```python
from build123d import *

# Parameters (mm, degrees)
CUT_EXTRUDE_1_DEPTH = 2


with BuildPart() as part:
    # 草图1 → 旋转1 (revolve)
    with BuildSketch(Plane.XY, mode=Mode.PRIVATE) as revolve_1_sk:
        Polygon((0, 14), (-3, 14), (-1.25, 12.25), (-1.25, 11.25), (-1.5, 11.25), (-1.5, 0), (0, 0), align=None)
    revolve(revolve_1_sk.sketch.rotate(Axis((0, 0, 0), (0, 1, 0)), 270), axis=Axis((0, 0, 0), (0, 1, 0)))

    # 草图2 → 切除-拉伸1 (cut)
    with BuildSketch(Plane(origin=(0, 14, 0), x_dir=(1, 0, 0), z_dir=(0, 1, 0))):
        Polygon((0.577350269, 1), (-0.577350269, 1), (-1.154700538, 0), (-0.577350269, -1), (0.577350269, -1), (1.154700538, 0), align=None)
    extrude(amount=-CUT_EXTRUDE_1_DEPTH, mode=Mode.SUBTRACT)


solid = part.part
```
Work out the finished part from the listing and answer in its coordinate system (mm). A direction names the side the tool comes from. Round coordinates to 2 decimals unless told otherwise and drop trailing zeros. Loops run counter-clockwise (first coordinate to the right, second up) from the corner with the lowest first, then second, coordinate; pieces in that order, holes last. Notation, with made-up numbers: (47.25, -13) -> (55.25, -13) arc R30 cw to (55.25, 19) -> close; hole circle Ø10 at (-33.5, 1.25). An arc over 180 degrees is marked (long way). Write each question's results on one line, items separated by ' | '. Start each with the question number.
1. For a pull along Z with two mould halves and no side action, classify faces 1 (the face through (-0.86, 13.01, -0.51)), 2 (the face through (-0.45, 5.55, -1.43)), 3 (the face through (0.86, 13.01, 0.51)), 4 (the face through (0, 0, 0)) as +Z half, -Z half, draft (parallel to the pull), parting line (faces both ways), or undercut.
2. A tool of negligible diameter and unlimited length cuts with its end or side. For faces 5 (the face through (1.22, 11.74, 0.27)), 6 (the face through (0, 14, 1.3)), 7 (the face through (0, 12, 0)), from which of +Z, -Z, +X, -X, +Y, -Y can it reach the whole face along a straight path? Write none if from no direction.
3. Section A-A (x = 0) is taken. Determine the outline of the cut face in (y, z).
4. Find the intervals of material crossed by probe 1 along Y at (x, z) = (-0.1, 0.1); probe 2 along Y at (x, z) = (1.5, -0.7); probe 3 along X at (y, z) = (3.5, 0.9), in increasing order. Write a range as from..to.
5. Section B-B (y = 9) is taken. Determine the outline of the cut face in (x, z), plus the area to 3 significant figures.
6. Given pin 1 Ø1.3 at (x, y) = (0.5, 13) entering from +Z; pin 2 Ø2 at (x, y) = (-0.5, 9) entering from -Z, each flat-ended and moving along its own axis, determine where each tip first touches the part or whether it passes through.
Evaluation:
1) face 1: undercut | face 2: parting line | face 3: undercut | face 4: draft
2) face 5: none | face 6: +Z, -Z, +X, -X, +Y | face 7: +Y
3) outline: (0, -1.5) -> (11.25, -1.5) -> (11.25, -1.25) -> (12.25, -1.25) -> (14, -3) -> (14, -1) -> (12, -1) -> (12, 1) -> (14, 1) -> (14, 3) -> (12.25, 1.25) -> (11.25, 1.25) -> (11.25, 1.5) -> (0, 1.5) -> close
4) probe 1: y = 0..12 | probe 2: y = 12.66..14 | probe 3: x = -1.2..1.2
5) outline: circle Ø3 at (0, 0) | area: 7.07 mm2
6) pin 1: stops at z = 2.61 | pin 2: stops at z = -1.5
